Autodesk Fusion 360 part; units mm, degrees
sketch "Sketch1" plane through (0, 0, 0) normal (1, 0, 0) x (0, 0, -1)
  line L0 (0, 0) -> (0, 40)
  line L1 (0, 40) -> (18, 40)
  line L2 (18, 40) -> (60, 30.6888)
  line L3 (0, 0) -> (60, 0)
  line L4 (60, 0) -> (60, 30.6888)
  dimension "d1" = 40
  dimension "d2" = 18
  dimension "d3" = 12.5
  dimension "d4" = 60
extrude "Extrude1" add sketch "Sketch1" along normal blind 50 makes body 1
sketch "Sketch2" plane through (0, 0, 0) normal (-1, 0, 0) x (0, 0, 1)
  line L0 (-60, 0) -> (0, 0)
  line L1 (0, 0) -> (0, 40)
  line L2 (0, 40) -> (-18, 40)
  line L3 (-18, 40) -> (-60, 30.6888)
  line L4 (-60, 30.6888) -> (-60, 0)
  circle A0 centre (-47.5, 20) radius 4.25
  line L5 (-60, 20) -> (0, 20) construction
  circle A1 centre (-12.5, 20) radius 4.25
  circle A2 centre (-47.5, 20) radius 7.25
  circle A3 centre (-12.5, 20) radius 7.25
  dimension "d9" = 8.5
  dimension "d12" = 12.5
  dimension "d13" = 12.5
  dimension "d14" = 14.5
  dimension "d15" = 20
extrude "Extrude2" cut sketch "Sketch2" against normal blind 63 contours A0 | A1 bodies 1
fillet "Fillet1" radius 57.5 1 edges at (25, 40, -18) on bodies 1
fillet "Fillet1" radius 3 4 edges at (25, 30.6888, -60) (25, 40, 0) (25, 0, 0) (25, 0, -60) on bodies 1
chamfer "Chamfer1" distance 0.4 angle 45 2 faces at (16.6667, 19.5768, -8.2711) (16.6667, 19.5768, -43.2711) on bodies 1
chamfer "Chamfer1" distance 2 angle 45 10 faces at (16.6667, 36.1613, -35.3151) (16.6667, 28.9517, -59.9241) (33.3333, 11.427, -60) (16.6667, 1.1455, -59.3582) (33.3333, 0, -21) (16.6667, 0.0034, -2.8573) (16.6667, 14.3333, 0) (16.6667, 38.3747, -0.3335) (16.6667, 40, -5.9009) (16.6667, 39.5782, -18.6549) on bodies 1
copy_body "Body->Comp1" bodies 1 removing the originals makes body 2 in component "bumper block"
component "bumper block" placed x (1, 0, 0) y (0, 1, 0) z (0, 0, 1) at (0, 0, 0)
The model under review builds one solid part; all positions refer to its coordinate system, in mm. Round coordinates to 2 decimals unless told otherwise and drop trailing zeros. Loops run counter-clockwise (first coordinate to the right, second up) from the corner with the lowest first, then second, coordinate; pieces in that order, holes last. Notation, with made-up numbers: (-25, -4) -> (-10, -4) arc R23 ccw to (-10, 14) -> close; hole circle Ø7 at (44.5, -31). An arc over 180 degrees is marked (long way). Answer as CSV lines item,"result".
1) Add section B-B on y = 20. Write out the cut boundary in (x, z), plus the area to 3 significant figures.
Geometry results:
outline,"(0, -58) -> (2, -60) -> (48, -60) -> (50, -58) -> (50, -52.15) -> (49.6, -51.75) -> (0.4, -51.75) -> (0, -52.15) -> close; (0, -42.85) -> (0.4, -43.25) -> (49.6, -43.25) -> (50, -42.85) -> (50, -17.15) -> (49.6, -16.75) -> (0.4, -16.75) -> (0, -17.15) -> close; (0, -7.85) -> (0.4, -8.25) -> (49.6, -8.25) -> (50, -7.85) -> (50, -2) -> (48, 0) -> (2, 0) -> (0, -2) -> close"
area,"2,140 mm²"
2) Draft analysis for pull direction Y (two halves, no side actions). For faces 1 (the face through (49, 15, -59)), 2 (the face through (48.986, 1.592, -58.44)), 3 (the face through (48.986, 38.687, -17.769)), state which applies: pulls with the +Y half, pulls with the -Y half, needs draft (parallel to the pull), parting line crosses it, or undercut.
Geometry results:
face 1,"needs draft"
face 2,"pulls with the -Y half"
face 3,"pulls with the +Y half"
3) Add section C-C on z = -47.5. Write out the cut boundary in (x, y).
Geometry results:
outline,"(0, 2) -> (2, 0) -> (48, 0) -> (50, 2) -> (50, 15.35) -> (49.6, 15.75) -> (0.4, 15.75) -> (0, 15.35) -> close; (0, 24.65) -> (0.4, 24.25) -> (49.6, 24.25) -> (50, 24.65) -> (50, 31.41) -> (48, 33.46) -> (2, 33.46) -> (0, 31.41) -> close"
4) Add section D-D on z = -29. Write out the cut boundary in (x, y).
Geometry results:
outline,"(0, 2) -> (2, 0) -> (48, 0) -> (50, 2) -> (50, 35.51) -> (48, 37.56) -> (2, 37.56) -> (0, 35.51) -> close"
5) For P1, Ø8, axis at x = 19, z = -18.5, coming from the +Y side; P2, Ø1, axis at x = 34, z = -17.5, coming from the +Y side; P3, Ø5, axis at y = 20, z = -12.5, coming from the +X side; P4, Ø10, axis at x = 16, y = 33.5, coming from the -Z side, all flat-tipped, find the tip position at first contact; note any pin that passes through.
Geometry results:
P1,"stops at y = 39.93"
P2,"stops at y = 39.76"
P3,"passes through"
P4,"stops at z = -59.99"
6) To check wall thickness, follow line 1 along Z through (x, y) = (20, 20.5); line 2 along Z through (x, y) = (29, 18.5); line 3 along Y through (x, z) = (33, -12.5). State the ranges of each line that lie inside material, in increasing order. Write a range as from..to.
Geometry results:
line 1,"z = -60..-51.72, -43.28..-16.72, -8.28..0"
line 2,"z = -60..-51.48, -43.52..-16.48, -8.52..0"
line 3,"y = 0..15.75, 24.25..39.99"
7) Add section A-A on x = 3.5. Write out the cut boundary in (y, z).
Geometry results:
outline,"(0, -57) arc R3 ccw to (3, -60) -> (28.28, -60) arc R3 ccw to (31.21, -57.65) -> (38.64, -24.15) arc R57.5 ccw to (40, -11.7) -> (40, -3) arc R3 ccw to (37, 0) -> (3, 0) arc R3 ccw to (0, -3) -> close; hole circle Ø8.5 at (20, -47.5); hole circle Ø8.5 at (20, -12.5)"
